from build123d import *

# Parameters (mm, degrees)
F0_W     = 304.8
F0_H     = 152.4
F1_DEPTH = 76.2
F2_T     = -6.35
F3_R     = 6.35
F4_DEPTH = 434.16217
F5_R     = 6.35
F6_DEPTH = 64.02061


with BuildPart() as f1:
    # F0 (on Front) → F1 (new body, symmetric)
    with BuildSketch(Plane.XZ):
        Rectangle(F0_W, F0_H)
    extrude(amount=F1_DEPTH, both=True)

    # F2
    f2_openings = [f1.faces().sort_by_distance(p)[0] for p in [
        (0, 0, -76.2),
    ]]
    offset(amount=F2_T, openings=f2_openings)

    # F3 (on face) → F4 (cut)
    with BuildSketch(Plane.YZ.offset(152.4)):
        Circle(F3_R)
    extrude(amount=-F4_DEPTH, mode=Mode.SUBTRACT)

    # F5 (on face) → F6 (cut)
    with BuildSketch(Plane.XY.offset(76.2)):
        with Locations((-38.1, 0)):
            Circle(F5_R)
        with Locations((38.1, 0)):
            Circle(F5_R)
    extrude(amount=-F6_DEPTH, mode=Mode.SUBTRACT)


solid = f1.part
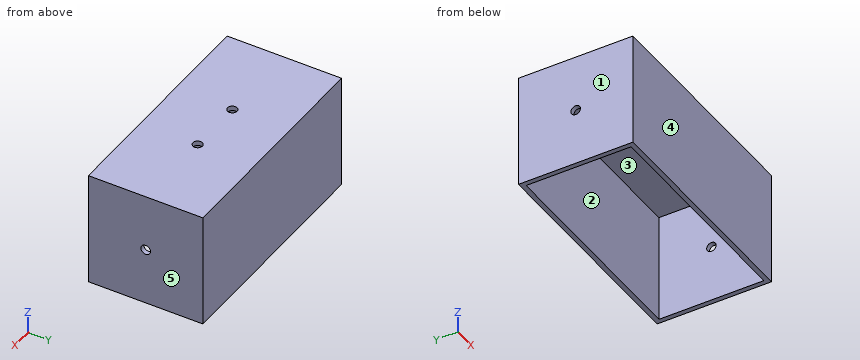
CAD build for the part. Positions are in the model's coordinates, mm. Face numbers are marked on the shaded views. A direction names the side the tool comes from. Round coordinates to 2 decimals unless told otherwise and drop trailing zeros. Write each loop counter-clockwise with the first axis right and the second up, starting at its lowest first coordinate (ties: lowest second). Pieces come first, ordered by that corner, then holes.
(1) 3-axis set-ups, long thin cutter, end or side, ignore diameter. For the marked faces 1 and 2: which of +Z, -Z, +X, -X, +Y, -Y reach the whole face in a straight line?
(2) Drop a flat-ended pin along its axis: P1, Ø2, axis at x = -96.5, y = -6, coming from the -Z side. Give the stop position or say it passes through.
(3) Mould opens along X. For the marked faces 3, 4 and 5 say: pulls with the +X half, pulls with the -X half, needs draft (parallel to the pull), parting line crosses it, or undercut.
(4) Slice it at C-C, the plane z = -37.5. Write the cut outline in (x, y).
(5) Slice it at A-A, the plane y = 0. Write the cut outline in (x, z).
(6) Slice it at D-D, the plane x = -91.5. Write the cut outline in (y, z), and give its area (3 significant figures).
(7) Probe line 1 along X through (y, z) = (-20, -4); line 2 along Z through (x, y) = (-149.5, 0). List the from-to ranges inside material, lowest first.
(8) Slice it at B-B, the plane x = -38.1. Write the cut outline in (y, z).
From the geometry:
1. face 1: +Z, -Z, -X, +Y, -Y
1. face 2: -Z
2. P1: stops at z = 69.85
3. face 3: undercut
3. face 4: needs draft
3. face 5: pulls with the +X half
4. outline: (-152.4, -76.2) - (152.4, -76.2) - (152.4, 76.2) - (-152.4, 76.2) - close; hole (-146.05, -69.85) - (146.05, -69.85) - (146.05, 69.85) - (-146.05, 69.85) - close
5. outline: (-152.4, -76.2) - (-146.05, -76.2) - (-146.05, -6.35) - (-152.4, -6.35) - close; (-152.4, 6.35) - (-146.05, 6.35) - (-146.05, 69.85) - (-44.45, 69.85) - (-44.45, 76.2) - (-152.4, 76.2) - close; (-31.75, 69.85) - (31.75, 69.85) - (31.75, 76.2) - (-31.75, 76.2) - close; (44.45, 69.85) - (146.05, 69.85) - (146.05, 6.35) - (152.4, 6.35) - (152.4, 76.2) - (44.45, 76.2) - close; (146.05, -76.2) - (152.4, -76.2) - (152.4, -6.35) - (146.05, -6.35) - close
6. outline: (-76.2, -76.2) - (-69.85, -76.2) - (-69.85, 69.85) - (69.85, 69.85) - (69.85, -76.2) - (76.2, -76.2) - (76.2, 76.2) - (-76.2, 76.2) - close
6. area: 2,820 mm2
7. line 1: x = -152.4 to -146.05, 146.05 to 152.4
7. line 2: z = -76.2 to -6.35, 6.35 to 76.2
8. outline: (-76.2, -76.2) - (-69.85, -76.2) - (-69.85, 69.85) - (-6.35, 69.85) - (-6.35, 76.2) - (-76.2, 76.2) - close; (6.35, 69.85) - (69.85, 69.85) - (69.85, -76.2) - (76.2, -76.2) - (76.2, 76.2) - (6.35, 76.2) - close
